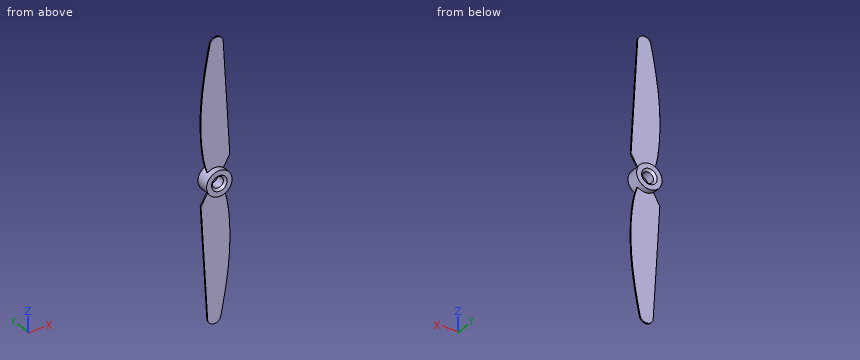
Autodesk Fusion 360 part; units mm, degrees
sketch "Sketch1" plane through (0, 0, 0) normal (0, 1, 0) x (1, 0, 0)
  circle A0 centre (0, 0) radius 5.75
  dimension "d1" = 11.5
extrude "Extrude1" add sketch "Sketch1" along normal mid plane 6
sketch "Sketch2" plane through (0, 0, 0) normal (0, 0, 1) x (1, 0, 0)
  line L0 (5.75, 3) -> (-5.75, 3)
  line L1 (-5.75, -3) -> (5.75, -3)
  line L2 (-5.99, 1.3829) -> (5.9749, -1.3794)
  dimension "d4" = 13
sketch "Sketch3" plane through (0, 0, 0) normal (0, 1, 0) x (1, 0, 0)
  circle A0 centre (0, 0) radius 5.75
  line L0 (-3.5598, 4.5155) -> (-6.478, 9.5938)
  line L1 (-6.478, 9.5938) -> (-3.4813, 60.953)
  spline S0 degree 5 poles (3.5598, 4.5155) (3.6773, 4.794) (3.9082, 5.3773) (4.2425, 6.332) (4.664, 7.7653) (5.1484, 9.8443) (5.5861, 12.2602) (5.9693, 15.1008) (6.2849, 18.4604) (6.5067, 22.3972) (6.6011, 26.9122) (6.5015, 31.8707) (6.167, 37.0685) (5.6191, 42.3359) (4.9052, 47.5085) (4.0907, 52.4479) (3.4107, 56.1235) (2.9079, 58.6916) (2.5788, 60.3158) (2.4158, 61.106) knots 0 0 0 0 0 0 0.066667 0.133333 0.2 0.266667 0.333333 0.4 0.466667 0.533333 0.6 0.666667 0.733333 0.8 0.866667 0.933333 1 1 1 1 1 1
  line L2 (-2.2481, 63.5) -> (-1.4613, 63.5)
  arc A1 (2.4158, 61.106) -> (-3.4633, 61.0922) centre (-0.5223, 60.5) ccw
  arc A2 (-3.4633, 61.0922) -> (-3.4813, 60.953) centre (-2.483, 60.8948) ccw
  line L3 (-3.5598, 4.5155) -> (3.5598, 4.5155) construction
  line L4 (6.5565, 20.5742) -> (6.5493, 33.2506)
  point P0 (5.1258, 9.8758)
  point P1 (6.5529, 26.9124)
  dimension "d5" = 3
  dimension "d6" = 1
  dimension "d7" = 63.5
  dimension "d9" = 12
extrude "Extrude2" add sketch "Sketch3" along normal mid plane 0.6 contours A0 L0 L1 S0 A1 A2
pattern_circular "C-Pattern1" count 2 over 360 about axis through (0, 1.75, 0) along (0, 1, 0) of "Extrude2"
sketch "Sketch4" plane through (0, 3, 0) normal (0, 1, 0) x (-1, 0, 0)
  circle A0 centre (0, 0) radius 5.75
  circle A1 centre (0, 0) radius 2.5
  dimension "d16" = 5
extrude "Extrude3" cut sketch "Sketch4" against normal blind 16 contours A1
chamfer "Chamfer1" distance 1 angle 45 2 edges at (2.3308, 3, 0.904) (2.3308, -3, -0.904)
Geometry check sheet. Reference: the model listing, model coordinates, mm. Give positions to 0.01 mm unless a question says otherwise; leave off trailing zeros. Order: outer loops, then holes, each group sorted by start corner. A loop starts at its lowest first (then second) coordinate and runs counter-clockwise, first axis right, second up.
1. Section check A-A, the plane z = 0. Enter the section's corners in (x, y), and give its area (3 significant figures).
2. Thickness scan on L1, parallel to Z at x = 0, y = 1; L2, parallel to Y at x = 1, z = 21; L3, parallel to Z at x = 2.25, y = -1.1. Record the ranges inside material, lowest first.
3. Section check B-B, the plane x = 0. Enter the section's corners in (y, z).
4. Gauge pin test, flat ends, axial feed: pin 1 Ø3 at (y, z) = (-1, 13.5) entering from +X; pin 2 Ø6.5 at (x, z) = (3, 45.5) entering from +Y; pin 3 Ø4 at (x, z) = (0, 0) entering from +Y; pin 4 Ø1 at (x, y) = (5, 1) entering from +Z. Record the tip position at first contact, or that the pin passes through.
Values follow:
1. outline: (-5.75, -3) - (-3.5, -3) - (-2.5, -2) - (-2.5, 2) - (-3.5, 3) - (-5.75, 3) - close; (2.5, -2) - (3.5, -3) - (5.75, -3) - (5.75, 3) - (3.5, 3) - (2.5, 2) - close
1. area: 37.0 mm2
2. L1: z = -5.75 to -2.5, 2.5 to 5.75
2. L2: y = -0.3 to 0.3
2. L3: z = -5.29 to -1.09, 1.09 to 5.29
3. outline: (-3, -5.75) - (-0.3, -5.75) - (-0.3, -63.45) - (0.3, -63.45) - (0.3, -5.75) - (3, -5.75) - (3, -3.5) - (2, -2.5) - (-2, -2.5) - (-3, -3.5) - close; (-3, 3.5) - (-2, 2.5) - (2, 2.5) - (3, 3.5) - (3, 5.75) - (0.3, 5.75) - (0.3, 63.45) - (-0.3, 63.45) - (-0.3, 5.75) - (-3, 5.75) - close
4. pin 1: stops at x = 6.33
4. pin 2: stops at y = 0.3
4. pin 3: passes through
4. pin 4: stops at z = 3.58
